```python
from build123d import *

# Parameters (mm, degrees)
SKETCH1_W                       = 9.525
SKETCH1_H                       = 76.2
BOSS_EXTRUDE1_DEPTH             = 28.575
F_10_24_TAPPED_HOLE1_AT_2_COUNT = 2
F_10_24_TAPPED_HOLE1_AT_2_PITCH = 34
FILLET1_R                       = 1.27


with BuildPart() as part:
    # Sketch1 → Boss-Extrude1 (new body, symmetric)
    with BuildSketch(Plane(origin=(0, 0, 0), x_dir=(1, 0, 0), z_dir=(0, 1, 0))):
        Rectangle(SKETCH1_W, SKETCH1_H)
    extrude(amount=BOSS_EXTRUDE1_DEPTH, both=True)

    # Sketch3 → #10-24 Tapped Hole1 (revolve, cut)
    with BuildSketch(Plane(origin=(0, 28.575, -17), x_dir=(0, 0, 1), z_dir=(1, 0, 0))):
        Polygon((0, 0), (0, 20.190824014), (1.89865, 19.05), (1.89865, 0), align=None)
    f_10_24_tapped_hole1 = revolve(axis=Axis((0, 34.925, -17), (0, -1, 0)), mode=Mode.SUBTRACT)

    # #10-24 Tapped Hole1 at 2: #10-24 Tapped Hole1 ×2
    with Locations(*[(0, 0, i * F_10_24_TAPPED_HOLE1_AT_2_PITCH) for i in range(1, F_10_24_TAPPED_HOLE1_AT_2_COUNT)]):
        add(f_10_24_tapped_hole1, mode=Mode.SUBTRACT)

    # Mirror1: #10-24 Tapped Hole1 across plane
    add(f_10_24_tapped_hole1.mirror(Plane.ZX), mode=Mode.SUBTRACT)

    # Mirror1 copy 1 sketch → Mirror1 copy 1 (revolve, cut)
    with BuildSketch(Plane(origin=(0, -28.575, 17), x_dir=(0, 0, 1), z_dir=(1, 0, 0))):
        Polygon((0, 0), (0, -20.190824014), (1.89865, -19.05), (1.89865, 0), align=None)
    revolve(axis=Axis((0, -34.925, 17), (0, -1, 0)), mode=Mode.SUBTRACT)

    # Fillet1
    fillet1_edges = [part.edges().sort_by_distance(p)[0] for p in [
        (-4.7625, 0, -38.1),
        (4.7625, 0, -38.1),
        (4.7625, 0, 38.1),
        (-4.7625, 0, 38.1),
    ]]
    fillet(fillet1_edges, radius=FILLET1_R)


solid = part.part
```
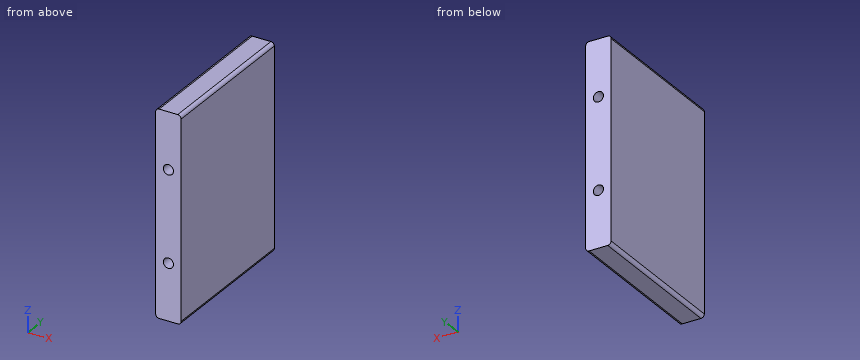
Can you work these out from the model? Positions are in its coordinate system, mm. Round coordinates to 2 decimals unless told otherwise and drop trailing zeros. Loops run counter-clockwise (first coordinate to the right, second up) from the corner with the lowest first, then second, coordinate; pieces in that order, holes last. Notation, with made-up numbers: M -21,88.5 L 7,88.5 A36 cw 7,127.5 Z; hole C -20,40 d2. An arc over 180 degrees is marked long. Answer as a JSON object with one key per item and string values. Group by question number.
Q1. Will this pin go through, and if not, where does the flat tip stop? pin 1 (3.5 mm diameter, centred on x = 0, z = 17, fed in from +Y).
Q2. Imagine slicing it at A-A, the plane y = -12. Please give me the cut outline in (x, z).
Q3. Please list where these lines run through material, in increasing order: L1, parallel to Z at x = 0, y = -22.5; L2, parallel to X at y = -22, z = 17; L3, parallel to Z at x = 4, y = 0.5.
Findings:
{
 "1": {"pin 1": "stops at y = 9.44"},
 "2": {"outline": "M -4.76,-36.83 A1.27 ccw -3.49,-38.1 L 3.49,-38.1 A1.27 ccw 4.76,-36.83 L 4.76,36.83 A1.27 ccw 3.49,38.1 L -3.49,38.1 A1.27 ccw -4.76,36.83 Z; hole C 0,-17 d3.8; hole C 0,17 d3.8"},
 "3": {"L1": "z = -38.1 to -18.9, -15.1 to 15.1, 18.9 to 38.1", "L2": "x = -4.76 to -1.9, 1.9 to 4.76", "L3": "z = -37.99 to 37.99"}
}
